Autodesk Inventor part; units mm, degrees
ref_plane "YZ Plane" through (0, 0, 0) normal (1, 0, 0) x (0, 1, 0)
ref_plane "XZ Plane" through (0, 0, 0) normal (0, 1, 0) x (-1, 0, 0)
ref_plane "XY Plane" through (0, 0, 0) normal (0, 0, 1) x (1, 0, 0)
sketch "Sketch1" plane through (0, 0, 0) normal (0, 1, 0) x (-1, 0, 0)
  line L0 (-32.512, -44.196) -> (32.512, -44.196)
  line L1 (32.512, -44.196) -> (32.512, 44.196)
  line L2 (32.512, 44.196) -> (-32.512, 44.196)
  line L3 (-32.512, 44.196) -> (-32.512, -44.196)
  line L4 (-32.512, -44.196) -> (32.512, 44.196) construction
  line L5 (32.512, -44.196) -> (-32.512, 44.196) construction
  point P0 (0, 0)
  point P1 (0, 0)
  dimension "d0" = 65.024
  dimension "d1" = 88.392
extrude "Extrusion1" add sketch "Sketch1" along normal blind 12.7
hole "Hole1" at (-25.4, 12.7, -37.084) direction (0, -1, 0) diameter 6.7564 end through all
hole "Hole3" at (25.4, 12.7, -37.084) direction (0, -1, 0) diameter 6.7564 end through all
hole "Hole4" at (25.4, 12.7, -11.684) direction (0, -1, 0) diameter 6.7564 end through all
hole "Hole5" at (25.4, 12.7, 13.716) direction (0, -1, 0) diameter 6.7564 end through all
hole "Hole6" at (0, 12.7, 13.716) direction (0, -1, 0) diameter 6.7564 end through all
hole "Hole7" at (-25.4, 12.7, 13.716) direction (0, -1, 0) diameter 6.7564 end through all
hole "Hole8" at (-25.4, 12.7, -11.684) direction (0, -1, 0) diameter 6.7564 end through all
sketch "Sketch2" plane through (0, 12.7, 0) normal (0, 1, 0) x (1, 0, 0)
  line L0 (-32.512, -44.5719) -> (32.512, -44.196)
  line L1 (32.512, -44.196) -> (25.4, -36.614)
  line L2 (25.4, -36.614) -> (-25.4, -36.614)
  line L3 (-25.4, -36.614) -> (-32.512, -44.5719)
  line L4 (-32.512, -44.5719) -> (25.4, -36.614) construction
  line L5 (32.512, -44.196) -> (-25.4, -36.614) construction
  point P0 (0, 0)
  point P1 (0.6144, -40.0199)
extrude "Extrusion2" add sketch "Sketch2" along normal blind 65.278
hole "Hole9" at (-0.0005, 52.578, 44.384) direction (-0.0057808, 0, -0.9999833) diameter 23.9268 end through all
sketch "Sketch3" plane through (32.512, 0, -44.196) normal (0, 0, -1) x (-1, 0, 0)
  line L0 (0, 12.7) -> (65.024, 12.7)
  line L1 (65.024, 12.7) -> (65.024, 0)
  line L2 (65.024, 0) -> (0, 0)
  line L3 (0, 0) -> (0, 12.7)
  line L4 (0, 12.7) -> (65.024, 0) construction
  line L5 (65.024, 12.7) -> (0, 0) construction
  point P0 (32.512, 0)
  point P1 (32.512, 6.35)
extrude "Extrusion3" add sketch "Sketch3" along normal blind 12.7
hole "Hole10" at (8.0772, 0, -45.166) direction (0, 1, 0) diameter 4.318 end through all counterbore diameter 7.112 counterbore depth 5.588
hole "Hole13" at (12.7, 12.7, 0.635) direction (0, -1, 0) diameter 4.9784 depth 7.62 tip angle 118
hole "Hole14" at (-12.7, 12.7, 0.635) direction (0, -1, 0) diameter 4.9784 depth 7.62 tip angle 118
sketch "Sketch4" plane through (32.512, 12.7, 36.614) normal (1, 0, 0) x (0, 0, -1)
  line L0 (-7.582, -12.7) -> (93.51, -12.7)
  line L1 (93.51, 0) -> (93.51, -12.7)
  line L2 (0, 0) -> (93.51, 0)
  line L3 (0, 0) -> (0, 65.278)
  line L4 (-7.582, 65.278) -> (0, 65.278)
  line L5 (-7.582, 0) -> (-7.582, 65.278)
  line L6 (-18.542, 0) -> (-18.1661, 0)
  line L7 (-7.582, -12.7) -> (-7.582, 0)
  point P0 (36.614, -12.7)
sketch "Sketch5" plane through (32.512, 12.7, 36.614) normal (1, 0, 0) x (0, 0, -1)
  line L0 (-7.582, -12.7) -> (93.51, -12.7)
  line L1 (93.51, 0) -> (93.51, -12.7)
  line L2 (0, 0) -> (93.51, 0)
  line L3 (0, 0) -> (0, 65.278)
  line L4 (-7.582, 65.278) -> (0, 65.278)
  line L5 (-7.582, 0) -> (-7.582, 65.278)
  line L6 (-18.542, 0) -> (-18.1661, 0)
  line L7 (-7.582, -12.7) -> (-7.582, 0)
  point P0 (36.614, -12.7)
sketch "Sketch6" plane through (0, 77.978, 0) normal (0, 1, 0) x (1, 0, 0)
  line L0 (-32.512, -44.5719) -> (32.512, -44.196)
  line L1 (32.512, -44.196) -> (25.4, -36.614)
  line L2 (25.4, -36.614) -> (-25.4, -36.614) construction
  line L3 (-25.4, -36.614) -> (-32.512, -44.5719)
  point P0 (0, 0)
sketch "Sketch7" plane through (32.512, 12.7, 36.614) normal (1, 0, 0) x (0, 0, -1)
  line L0 (-7.582, -12.7) -> (93.51, -12.7)
  line L1 (93.51, 0) -> (93.51, -12.7)
  line L2 (0, 0) -> (93.51, 0)
  line L3 (0, 0) -> (0, 65.278)
  line L4 (-7.582, 65.278) -> (0, 65.278)
  line L5 (-7.582, 0) -> (-7.582, 65.278) construction
  line L6 (-18.542, 0) -> (-18.1661, 0)
  line L7 (-7.582, -12.7) -> (-7.582, 0)
  point P0 (36.614, -12.7)
sketch "Sketch8" plane through (-32.512, 12.7, 44.5719) normal (0.0057808, 0, 0.9999833) x (0.9999833, 0, -0.0057808)
  circle A0 centre (32.512, 39.878) radius 11.9634
  line L0 (0, 0) -> (65.0251, 0)
  line L1 (65.0251, 0) -> (65.0251, 65.278)
  line L2 (0, 65.278) -> (65.0251, 65.278)
  line L3 (0, 0) -> (0, 65.278)
  point P0 (65.024, 0)
  point P1 (32.7691, -12.7)
hole "Hole16" at (12.7, 12.7, -24.765) direction (0, -1, 0) diameter 4.9784 depth 7.62 tip angle 118
hole "Hole17" at (-12.7, 12.7, -24.765) direction (0, -1, 0) diameter 4.9784 depth 7.62 tip angle 118
properties part number "DetectionAdapter"
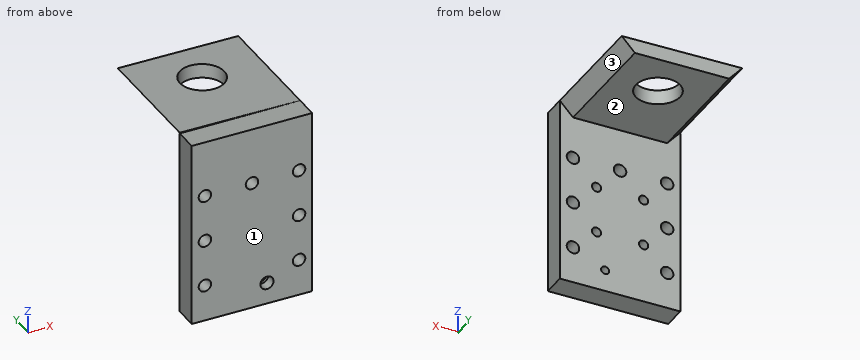
Model file for the job. Use its own axes, mm. Face numbers are marked on the shaded views. A direction names the side the tool comes from. Coordinates: 2 decimals unless noted, no trailing zeros. Loops run counter-clockwise (first coordinate to the right, second up) from the corner with the lowest first, then second, coordinate; pieces in that order, holes last. Notation, with made-up numbers: (13.25, -26) - (26.25, -26) arc R15 cw to (26.25, -19) - close; hole circle Ø4 at (61.5, 26.5). An arc over 180 degrees is marked (long way). Answer as a JSON object with one key per item and string values. Group by question number.
(1) Cut at B-B (z = -11.5). Give the cut face in (x, y), then the cut area to 3 significant figures.
(2) Flat gauge pins, fed straight in: pin 1 (7 mm diameter, centred on x = 8.08, z = -45.17, fed in from +Y); pin 2 (4 mm diameter, centred on x = 6.5, y = 5.5, fed in from +Z); pin 3 (12 mm diameter, centred on x = 6, y = 58.5, fed in from -Z). Where does each tip first touch, or does it go through?
(3) Cut at C-C (y = 28). Give the cut face in (x, z).
(4) Cut at A-A (y = 56). Give the cut face in (x, z), then the cut area to 3 significant figures.
(5) Probe line 1 along Z through (x, y) = (-25.4, 7.5); line 2 along Z through (x, y) = (0, 7.75); line 3 along Z through (x, y) = (12.7, 6.75). List the from-to ranges inside material, lowest first.
(6) Tool access for the marked faces 1, 2 and 3: list every direction of +Z, -Z, +X, -X, +Y, -Y with a clear straight run to the whole face (end or side of a thin tool).
Geometry says:
{
 "1": {"outline": "(-32.51, 0) - (-28.77, 0) - (-28.77, 12.7) - (-32.51, 12.7) - close; (-22.03, 0) - (22.03, 0) - (22.03, 12.7) - (-22.03, 12.7) - close; (28.77, 0) - (32.51, 0) - (32.51, 12.7) - (28.77, 12.7) - close", "area": "654 mm^2"},
 "2": {"pin 1": "stops at y = 12.7", "pin 2": "stops at z = 44.2", "pin 3": "stops at z = 36.61"},
 "3": {"outline": "(-32.51, 44.57) - (-25.4, 36.61) - (25.4, 36.61) - (32.51, 44.2) - close"},
 "4": {"outline": "(-32.51, 44.57) - (-25.4, 36.61) - (-11.51, 36.61) - (-11.46, 44.45) - close; (11.42, 36.61) - (25.4, 36.61) - (32.51, 44.2) - (11.46, 44.32) - close", "area": "272 mm^2"},
 "5": {"line 1": "z = -56.9 to -40.46, -33.71 to -15.06, -8.31 to 10.34, 17.09 to 44.2", "line 2": "z = -56.9 to 10.34, 17.09 to 44.2", "line 3": "z = -56.9 to -27.25, -22.28 to -1.85, 3.12 to 44.2"},
 "6": {"face 1": "+Z, -Z, +X, -X, -Y", "face 2": "-Z, +X, -X, +Y", "face 3": "-Z, +X, +Y"}
}
